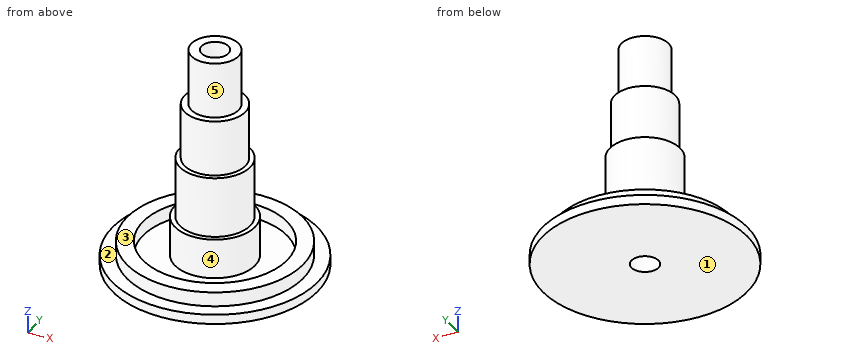
```python
from build123d import *

# Parameters (mm, degrees)
F0_R      = 64
F0_R_2    = 55
F1_DEPTH  = 6
F2_R      = 55
F2_R_2    = 45
F3_DEPTH  = 9
F4_R      = 25
F5_DEPTH  = 25
F6_R      = 22
F7_DEPTH  = 38
F8_R      = 19
F9_DEPTH  = 35
F10_R     = 14.75
F11_DEPTH = 35
F12_R     = 8.45
F13_DEPTH = 200


with BuildPart() as f1:
    # F0 (on Top) → F1 (new body)
    with BuildSketch(Plane.XY):
        Circle(F0_R)
        Circle(F0_R_2, mode=Mode.SUBTRACT)
        Circle(F0_R_2)
    extrude(amount=F1_DEPTH)

    # F2 (on face) → F3 (join)
    with BuildSketch(Plane.XY.offset(6)):
        Circle(F2_R)
        Circle(F2_R_2, mode=Mode.SUBTRACT)
    extrude(amount=F3_DEPTH)

    # F4 (on face) → F5 (join)
    with BuildSketch(Plane.XY.offset(6)):
        Circle(F4_R)
    extrude(amount=F5_DEPTH)

    # F6 (on face) → F7 (join)
    with BuildSketch(Plane.XY.offset(31)):
        Circle(F6_R)
    extrude(amount=F7_DEPTH)

    # F8 (on face) → F9 (join)
    with BuildSketch(Plane.XY.offset(69)):
        Circle(F8_R)
    extrude(amount=F9_DEPTH)

    # F10 (on face) → F11 (join)
    with BuildSketch(Plane.XY.offset(104)):
        Circle(F10_R)
    extrude(amount=F11_DEPTH)

    # F12 (on face) → F13 (cut)
    with BuildSketch(Plane.XY.offset(139)):
        Circle(F12_R)
    extrude(amount=-F13_DEPTH, mode=Mode.SUBTRACT)


solid = f1.part
```
Can you work these out from the model? Positions are in its coordinate system, mm. Face numbers are marked on the shaded views. A direction names the side the tool comes from. Coordinates: 2 decimals unless noted, no trailing zeros. Loops run counter-clockwise (first coordinate to the right, second up) from the corner with the lowest first, then second, coordinate; pieces in that order, holes last. Notation, with made-up numbers: (51, 69.25) - (64, 69.25) arc R8 ccw to (64, 73.25) - close; hole circle Ø3 at (-15.5, 76.25). An arc over 180 degrees is marked (long way). Use a Markdown table: item, result.
Item 1: For the marked faces 1 and 2, which set-ups out of +Z, -Z, +X, -X, +Y, -Y let a thin tool reach every point of the face, with its end or its side?
Numbers:
| item | result |
|---|---|
| face 1 | -Z, +X, -X, +Y, -Y |
| face 2 | +Z |
Item 2: If I drill on probe 1 along Y at (x, z) = (0, 10); probe 2 along Y at (x, z) = (0, 81); probe 3 along Y at (x, z) = (0, 41.5), over which ranges is the centre line in solid material (lowest first)? Write a range as from..to.
Numbers:
| item | result |
|---|---|
| probe 1 | y = -55..-45, -25..-8.45, 8.45..25, 45..55 |
| probe 2 | y = -19..-8.45, 8.45..19 |
| probe 3 | y = -22..-8.45, 8.45..22 |
Item 3: I want a section at C-C on z = 11.5. Please give me the cut outline in (x, y).
Numbers:
| item | result |
|---|---|
| outline | circle Ø110 at (0, 0); circle Ø50 at (0, 0); hole circle Ø90 at (0, 0); hole circle Ø16.9 at (0, 0) |
Item 4: Will these pins go through, and if not, where does the flat tip stop? pin 1 (3 mm diameter, centred on x = 28, z = 21, fed in from +Y); pin 2 (4 mm diameter, centred on x = -16.5, z = 20, fed in from -Y); pin 3 (12 mm diameter, centred on x = -1.5, y = 40, fed in from +Z); pin 4 (1.5 mm diameter, centred on y = 6.5, z = 102, fed in from +X).
Numbers:
| item | result |
|---|---|
| pin 1 | passes through |
| pin 2 | stops at y = -20.37 |
| pin 3 | stops at z = 15 |
| pin 4 | stops at x = 18.11 |
Item 5: We'd pull the mould along X, two halves only. Please class the marked faces 3, 4 and 5: released by +X, released by -X, zero draft, split by the parting line, or undercut.
Numbers:
| item | result |
|---|---|
| face 3 | zero draft |
| face 4 | undercut |
| face 5 | split by the parting line |
Item 6: I want a section at D-D on z = 100. Please give me the cut outline in (x, y), and give its area (3 significant figures).
Numbers:
| item | result |
|---|---|
| outline | circle Ø38 at (0, 0); hole circle Ø16.9 at (0, 0) |
| area | 910 mm2 |
